from build123d import *

# Parameters (mm, degrees)
SKETCH1_R               = 10
BOSS_EXTRUDE1_DEPTH     = 1
SKETCH2_R               = 10
BOSS_EXTRUDE2_DEPTH     = 3
BOSS_EXTRUDE2_TAPER     = 4
SKETCH3_R               = 9.790219564
BOSS_EXTRUDE3_DEPTH     = 2
BOSS_EXTRUDE3_TAPER     = 3
SKETCH4_R               = 9.685404006
BOSS_EXTRUDE4_DEPTH     = 3
BOSS_EXTRUDE4_TAPER     = 1
SKETCH5_R               = 9.633038811
BOSS_EXTRUDE5_DEPTH     = 14
CUT_EXTRUDE1_DEPTH      = 13
CUT_EXTRUDE1_DEPTH_BACK = 13
SKETCH6_W               = 17.15
SKETCH6_H               = 8
CUT_EXTRUDE2_DEPTH      = 13
CUT_EXTRUDE2_DEPTH_BACK = 13
SKETCH8_W               = 8
SKETCH8_H               = 8
CUT_EXTRUDE3_DEPTH      = 13
SKETCH9_R               = 1.25
CUT_EXTRUDE4_DEPTH      = 11
CHAMFER1_SIZE           = 2


with BuildPart() as part:
    # Sketch1 → Boss-Extrude1 (new body)
    with BuildSketch(Plane.XY):
        Circle(SKETCH1_R)
    extrude(amount=BOSS_EXTRUDE1_DEPTH)

    # Sketch2 → Boss-Extrude2 (add)
    with BuildSketch(Plane.XY.offset(1)):
        Circle(SKETCH2_R)
    extrude(amount=BOSS_EXTRUDE2_DEPTH, taper=BOSS_EXTRUDE2_TAPER)

    # Sketch3 → Boss-Extrude3 (add)
    with BuildSketch(Plane.XY.offset(4)):
        Circle(SKETCH3_R)
    extrude(amount=BOSS_EXTRUDE3_DEPTH, taper=BOSS_EXTRUDE3_TAPER)

    # Sketch4 → Boss-Extrude4 (add)
    with BuildSketch(Plane.XY.offset(6)):
        Circle(SKETCH4_R)
    extrude(amount=BOSS_EXTRUDE4_DEPTH, taper=BOSS_EXTRUDE4_TAPER)

    # Sketch5 → Boss-Extrude5 (add)
    with BuildSketch(Plane.XY.offset(9)):
        Circle(SKETCH5_R)
    extrude(amount=BOSS_EXTRUDE5_DEPTH)

    # Sketch6 → Cut-Extrude1 (cut, two sides: drawn at the far end of the back side and taken through both)
    with BuildSketch(Plane(origin=(0, 0, 0), x_dir=(0, 0, -1), z_dir=(1, 0, 0)).offset(-CUT_EXTRUDE1_DEPTH_BACK)):
        with Locations((-17.575, 0)):
            Rectangle(SKETCH6_W, SKETCH6_H)
    extrude(amount=CUT_EXTRUDE1_DEPTH + CUT_EXTRUDE1_DEPTH_BACK, mode=Mode.SUBTRACT)

    # Sketch7 → Cut-Extrude2 (cut, two sides: drawn at the far end of the back side and taken through both)
    with BuildSketch(Plane(origin=(0, 0, 0), x_dir=(1, 0, 0), z_dir=(0, 1, 0)).offset(-CUT_EXTRUDE2_DEPTH_BACK)):
        with BuildLine():
            Line((-8.763300561, -9), (-10.263300561, -9))
            Line((-10.263300561, -9), (-10.263300561, -28.451581468))
            Line((-10.263300561, -28.451581468), (9.633038811, -28.451581468))
            Line((9.633038811, -28.451581468), (9.633038811, -9))
            Line((9.633038811, -9), (4.716699439, -9))
            Line((4.716699439, -9), (4.388453733, -16.36))
            ThreePointArc((4.388453733, -16.36), (1.343744491, -21.139438677), (-4.008974444, -23))
            Line((-4.008974444, -23), (-8.178974444, -23))
            Line((-8.178974444, -23), (-8.763300561, -9))
        make_face()
    extrude(amount=CUT_EXTRUDE2_DEPTH + CUT_EXTRUDE2_DEPTH_BACK, mode=Mode.SUBTRACT)

    # Sketch8 → Cut-Extrude3 (cut)
    with BuildSketch(Plane(origin=(0, 0, 0), x_dir=(-1, 0, 0), z_dir=(0, 0, -1))):
        Rectangle(SKETCH8_W, SKETCH8_H)
    extrude(amount=-CUT_EXTRUDE3_DEPTH, mode=Mode.SUBTRACT)

    # Sketch9 → Cut-Extrude4 (cut, symmetric)
    with BuildSketch(Plane(origin=(0, 0, 0), x_dir=(1, 0, 0), z_dir=(0, 1, 0))):
        with Locations(Location((-3.763300561, -18, 0), (0, 0, 270))):
            Circle(SKETCH9_R)
    extrude(amount=CUT_EXTRUDE4_DEPTH, both=True, mode=Mode.SUBTRACT)

    # Chamfer1
    # the kernel refuses this chamfer: 2 mm, written as the material it takes off along each edge
    with BuildSketch(Plane(origin=(0, 0, 9), x_dir=(-0.022475112384337453, 0.9997474027589727, 0), z_dir=(-0.9997474027589727, -0.022475112384337453, 0))) as chamfer1_piece_1_section:
        Polygon((9.633038811 - CHAMFER1_SIZE, 0), (9.633038811 + CHAMFER1_SIZE * 0.0174524064372, CHAMFER1_SIZE * 0.999847695156), (9.633038811, 0), align=None)
    chamfer1_piece_1 = revolve(axis=Axis((0, 0, 9), (0, 0, -1)), revolution_arc=91.28783752, mode=Mode.PRIVATE)
    chamfer1_piece_1 = split(chamfer1_piece_1, bisect_by=Plane(origin=(4.752278324, 4.191519128, 8.202242122), z_dir=(0.9990069635270563, 0, 0.0445543131969368)), keep=Keep.TOP, mode=Mode.PRIVATE)
    add(chamfer1_piece_1, mode=Mode.SUBTRACT)
    with BuildSketch(Plane(origin=(0, 0, 9), x_dir=(1, 0, 0), z_dir=(0, 1, 0))) as chamfer1_piece_2_section:
        Polygon((9.633038811 - CHAMFER1_SIZE, 0), (9.633038811 + CHAMFER1_SIZE * 0.0174524064373, CHAMFER1_SIZE * 0.999847695156), (9.633038811, 0), align=None)
    chamfer1_piece_2 = revolve(axis=Axis((0, 0, 9), (0, 0, -1)), revolution_arc=91.28783752, mode=Mode.PRIVATE)
    chamfer1_piece_2 = split(chamfer1_piece_2, bisect_by=Plane(origin=(4.752278326, -4.191519128, 8.202242073), z_dir=(0.9990069635270563, 0, 0.0445543131969368)), keep=Keep.TOP, mode=Mode.PRIVATE)
    add(chamfer1_piece_2, mode=Mode.SUBTRACT)


solid = part.part
Here's how the part is built. I have some questions about the finished solid (model axes, mm). A direction names the side the tool comes from. Coordinates: 2 decimals unless noted, no trailing zeros. Order: outer loops, then holes, each group sorted by start corner. A loop starts at its lowest first (then second) coordinate and runs counter-clockwise, first axis right, second up. Notation, with made-up numbers: (38.25, 12) - (77.25, 12) arc R28 cw to (77.25, 31) - close; hole circle Ø11 at (74, 59.25). An arc over 180 degrees is marked (long way). Use CSV: the item, a comma, the result in double quotes. Start each with the question number.
1. Suppose I cut it at B-B on z = 7.75. List the corners of the cut face in (x, y) for me.
2. If we mould it in two halves opening along X, with no side actions, what happens to faces 1 (the face through (4, 0, 4)), 2 (the face through (-8.4, 4.4, 17.7)), 3 (the face through (-1.26, 9.63, 5.46))? For each: +X half, -X half, draft (parallel to the pull), parting line (faces both ways), or undercut.
3. Please list where these lines run through material, in increasing order: line 1 (Z direction, x = -8.25, y = -3.75); line 2 (X direction, y = 7, z = 18); line 3 (Y direction, x = 2.25, z = 6). Write a range as from..to.
4. For faces 4 (the face through (-2, -4, 12)), 5 (the face through (-3.095, -9.122, 15.902)), 6 (the face through (-7, 0, 9)), which set-ups out of +Z, -Z, +X, -X, +Y, -Y let a thin tool reach every point of the face, with its end or its side?
5. Suppose I cut it at D-D on x = -3.25. Give the number of separate pieces and of enclosed holes in the cut face, then the cut area to 3 significant figures.
6. I'm going to push flat-ended pins straight in: pin 1 (6.5 mm diameter, centred on x = 0.5, z = 7, fed in from -Y); pin 2 (3 mm diameter, centred on x = -3.76, z = 18, fed in from +Y); pin 3 (5 mm diameter, centred on x = -0.5, y = 0, fed in from +Z); pin 4 (6 mm diameter, centred on y = 3, z = 16.5, fed in from -X). Where does each tip first touch, or does it pass through?
7. Suppose I cut it at A-A on z = 10.75. List the corners of the cut face in (x, y) for me.
8. Suppose I cut it at C-C on z = 18.5. List the corners of the cut face in (x, y) for me.
Output:
1,outline,"(4.77, -8.39) - (4.77, -7.52) arc R8.91 ccw to (4.77, 7.52) - (4.77, 8.39) arc R9.65 ccw (long way) to start; hole (-4, -4) - (4, -4) - (4, 4) - (-4, 4) - close"
2,face 1,"undercut"
2,face 2,"-X half"
2,face 3,"parting line"
3,line 1,"z = 0..9"
3,line 2,"x = -6.62..-5.01, -2.51..3.82"
3,line 3,"y = -9.42..-4, 4..9.42"
4,face 4,"+Z"
4,face 5,"+Z, -Y"
4,face 6,"+Z, +X, -X"
5,separate pieces,"4"
5,enclosed holes,"0"
5,area,"213 mm2"
6,pin 1,"stops at y = -9.81"
6,pin 2,"stops at y = 9.36"
6,pin 3,"passes through"
6,pin 4,"stops at x = -8.57"
7,outline,"(-8.69, -4.16) arc R9.63 ccw to (4.64, -8.44) - (4.64, -4) - (-8.69, -4) - close; (-8.69, 4) - (4.64, 4) - (4.64, 8.44) arc R9.63 ccw to (-8.69, 4.16) - close"
8,outline,"(-8.37, -4.77) arc R9.63 ccw to (-4.91, -8.29) - (-4.91, -4) - (-8.37, -4) - close; (-8.37, 4) - (-4.91, 4) - (-4.91, 8.29) arc R9.63 ccw to (-8.37, 4.77) - close; (-2.62, -9.27) arc R9.63 ccw to (3.57, -8.95) - (3.57, -4) - (-2.62, -4) - close; (-2.62, 4) - (3.57, 4) - (3.57, 8.95) arc R9.63 ccw to (-2.62, 9.27) - close"
